Part model, mm, in its own coordinate system. A direction names the side the tool comes from. Round coordinates to 2 decimals unless told otherwise and drop trailing zeros. Loops run counter-clockwise (first coordinate to the right, second up) from the corner with the lowest first, then second, coordinate; pieces in that order, holes last. Notation, with made-up numbers: (-1.5, 42.5) -> (8.5, 42.5) arc R26 cw to (8.5, 59.5) -> close; hole circle Ø5 at (-34, 6.25). An arc over 180 degrees is marked (long way). Use a Markdown table: item, result. Add a question column.
Item 1: Two-plate mould, pull along X, no slides. Class faces 3 (the face through (60, -15, 15)), 4 (the face through (17.3, -10.8, 18.5)), 5 (the face through (52, -20, 25)): pulls with the +X half, pulls with the -X half, needs draft (parallel to the pull), parting line crosses it, or undercut.
Item 2: Cut at D-D, the plane z = 16. List the corners of the cut face in (x, y).
Item 3: Cut at C-C, the plane x = 12. List the corners of the cut face in (y, z), plus the area to 3 significant figures.
Item 4: Which spindle directions (+Z, -Z, +X, -X, +Y, -Y) get a long thin tool onto all of the face, cutting with end or side? Do faces 1 (the face through (30, -40, 5)), 2 (the face through (30, -24, 10)). Say none if no direction does.
Item 5: Cut at B-B, the plane y = -30. List the corners of the cut face in (x, z), plus the area to 4 significant figures.
Item 6: Flat gauge pins, fed straight in: pin 1 (8 mm diameter, centred on y = -10.5, z = 28.5, fed in from -X); pin 2 (3 mm diameter, centred on x = 37.5, y = -17.5, fed in from +Z). Where does each tip first touch, or does it go through?
Item 7: Cut at A-A, the plane z = 26.5. List the corners of the cut face in (x, y), plus the area to 3 significant figures.
Item 8: Probe line 1 (Z direction, x = 17.5, y = -35.5); line 2 (X direction, y = -17.5, z = 20) (3 decimals); line 3 (X direction, y = -22, z = 22.5). List the from-to ranges inside material, lowest first. Write a range as [from, to].
```python
from build123d import *

# Parameters (mm, degrees)
F0_W     = 60
F0_H     = 40
F1_DEPTH = 40
F3_DEPTH = 30
F5_DEPTH = 30
F7_DEPTH = 20
F9_DEPTH = 20


with BuildPart() as f1:
    # F0 (on Front) → F1 (new body)
    with BuildSketch(Plane.XZ):
        with Locations((30, 20)):
            Rectangle(F0_W, F0_H)
    extrude(amount=F1_DEPTH)

    # F2 (on face) → F3 (cut)
    with BuildSketch(Plane.XY.offset(40)):
        Polygon((30, 0), (30, -40), (50, -40), (40, 0), align=None)
    extrude(amount=-F3_DEPTH, mode=Mode.SUBTRACT)

    # F4 (on face) → F5 (cut)
    with BuildSketch(Plane.XY.offset(40)):
        Polygon((30, -40), (30, 0), (20, 0), (10, -40), align=None)
    extrude(amount=-F5_DEPTH, mode=Mode.SUBTRACT)

    # F6 (on face) → F7 (cut)
    with BuildSketch(Plane.YZ.offset(60)):
        Polygon((-40, 10), (0, 40), (-40, 40), align=None)
    extrude(amount=-F7_DEPTH, mode=Mode.SUBTRACT)

    # F8 (on face) → F9 (cut)
    with BuildSketch(Plane(origin=(0, 0, 0), x_dir=(0, -1, 0), z_dir=(-1, 0, 0))):
        Polygon((40, 40), (0, 40), (40, 10), align=None)
    extrude(amount=-F9_DEPTH, mode=Mode.SUBTRACT)


solid = f1.part
```
A:
| question | item | result |
|---|---|---|
| 1 | face 3 | pulls with the +X half |
| 1 | face 4 | undercut |
| 1 | face 5 | needs draft |
| 2 | outline | (0, -32) -> (12, -32) -> (20, 0) -> (0, 0) -> close; (40, 0) -> (48, -32) -> (60, -32) -> (60, 0) -> close |
| 3 | outline | (-40, 0) -> (0, 0) -> (0, 40) -> (-32, 16) -> (-32, 10) -> (-40, 10) -> close |
| 3 | area | 976 mm^2 |
| 4 | face 1 | +Z, -Z, +X, -X, -Y |
| 4 | face 2 | +Z, -Y |
| 5 | outline | (0, 0) -> (60, 0) -> (60, 17.5) -> (47.5, 17.5) -> (47.5, 10) -> (12.5, 10) -> (12.5, 17.5) -> (0, 17.5) -> close |
| 5 | area | 787.5 mm^2 |
| 6 | pin 1 | stops at x = 0 |
| 6 | pin 2 | stops at z = 10 |
| 7 | outline | (0, -18) -> (15.5, -18) -> (20, 0) -> (0, 0) -> close; (40, 0) -> (44.5, -18) -> (60, -18) -> (60, 0) -> close |
| 7 | area | 639 mm^2 |
| 8 | line 1 | z = [0, 10] |
| 8 | line 2 | x = [0, 15.625], [44.375, 60] |
| 8 | line 3 | x = [0, 14.5], [45.5, 60] |
